```python
from build123d import *

# Parameters (mm, degrees)
F0_W     = 22
F0_H     = 35
F0_R     = 8
F1_DEPTH = 7.5
F3_DEPTH = 2
F6_DEPTH = 5
F7_R     = 2
F8_DEPTH = 35.001
F9_R     = 2.99999


# Not quite as in the source:
# - a fillet or chamfer is up to 0.001 mm smaller than in the source, because OpenCascade refuses the exact size


with BuildPart() as f1:
    # F0 (on Front) → F1 (new body, symmetric)
    with BuildSketch(Plane.XZ):
        with Locations((0, -2.5)):
            Rectangle(F0_W, F0_H)
        Circle(F0_R, mode=Mode.SUBTRACT)
    extrude(amount=F1_DEPTH, both=True)

    # F2 (on face) → F3 (cut)
    with BuildSketch(Plane(origin=(0, 0, -20), x_dir=(1, 0, 0), z_dir=(0, 0, -1))):
        with BuildLine():
            Line((2.5, 7.5), (-2.5, 7.5))
            Line((-2.5, 7.5), (-2.5, 2.5583377574))
            ThreePointArc((-2.5, 2.5583377574), (0, -3.5770227957), (2.5, 2.5583377574))
            Line((2.5, 2.5583377574), (2.5, 7.5))
        make_face()
    extrude(amount=-F3_DEPTH, mode=Mode.SUBTRACT)

    # F5 (on offset) → F6 (cut)
    with BuildSketch(Plane(origin=(0, 0, -18), x_dir=(1, 0, 0), z_dir=(0, 0, -1))):
        with BuildLine():
            Line((5, 7.5), (-5, 7.5))
            Line((-5, 7.5), (-5, 2.5583377574))
            ThreePointArc((-5, 2.5583377574), (0, -5.6165017654), (5, 2.5583377574))
            Line((5, 2.5583377574), (5, 7.5))
        make_face()
    extrude(amount=-F6_DEPTH, mode=Mode.SUBTRACT)

    # F7 (on face) → F8 (cut, through all)
    with BuildSketch(Plane.XY.offset(15)):
        Circle(F7_R)
    extrude(amount=-F8_DEPTH, mode=Mode.SUBTRACT)

    # F9 (radius 3 in the source; OpenCascade refuses exactly that, so slightly less here)
    f9_edges = [f1.edges().sort_by_distance(p)[0] for p in [
        (-11, 0, 15),
        (11, 0, 15),
        (0, -7.5, 15),
        (0, 7.5, 15),
        (11, -7.5, -2.5),
        (-11, -7.5, -2.5),
        (-11, 7.5, -2.5),
        (11, 7.5, -2.5),
        (0, 7.5, -20),
        (-6.75, -7.5, -20),
        (6.75, -7.5, -20),
        (-11, 0, -20),
        (11, 0, -20),
    ]]
    fillet(f9_edges, radius=F9_R)


solid = f1.part
```
Input: part model. Units: mm. Frame: model coordinates. A direction names the side the tool comes from. Give positions to 0.01 mm unless a question says otherwise; leave off trailing zeros. Order: outer loops, then holes, each group sorted by start corner. A loop starts at its lowest first (then second) coordinate and runs counter-clockwise, first axis right, second up. Notation, with made-up numbers: M 81,-34 L 93,-34 A20 ccw 93,-3 Z; hole C -3.75,1 d4. An arc over 180 degrees is marked long. One line per question, with ' | ' between items. Start each with the question number.
1. First-contact query: pin 1 Ø2 at (y, z) = (-4, -19.5) entering from +X; pin 2 Ø2.5 at (x, y) = (0, 0) entering from -Z; pin 3 Ø1 at (y, z) = (-4, -18.5) entering from -X; pin 4 Ø4.5 at (x, y) = (0, 0) entering from -Z. Flat tips, straight axial feed; report the tip coordinate or a pass-through.
2. Section query B-B (x = 0). Return the cut outline in (y, z).
3. Access query for faces 1 (the face through (5.29, -6.6, -19.14)), 2 (the face through (-0.161, 5.614, -15.535)), 3 (the face through (-2.5, -4, -19)), 4 (the face through (-0.119, 3.575, -19.014)). Directions: +Z, -Z, +X, -X, +Y, -Y. A direction counts if a zero-diameter tool reaches every point of the face in a straight line with its end or side. Return the directions, or none.
4. Pull-direction query (Z, two-part tool) for faces 5 (the face through (0, 7.5, -9)), 6 (the face through (-10.14, -0.06, -19.1)), 7 (the face through (-0.1, -2.5, -13)); classes: released by +Z, released by -Z, zero draft, split by the parting line, or undercut.
5. Section query C-C (y = 0). Return the cut outline in (x, z), and give its area (3 significant figures).
6. Material intervals for probe 1 along Y at (x, z) = (0, 10.5); probe 2 along Z at (x, y) = (3.5, 2.25); probe 3 along Z at (x, y) = (0, -3.5), sorted ascending. Write a range as [from, to].
7. Section query D-D (z = -12). Return the cut outline in (x, y), and give its area (3 significant figures).
Here are the results:
1) pin 1: x = 10.6 | pin 2: through | pin 3: x = -10.83 | pin 4: z = -13
2) outline: M -7.5,-13 L -2,-13 L -2,-8 L -7.5,-8 Z; M -7.5,8 L -2,8 L -2,15 L -4.5,15 A3 ccw -7.5,12 Z; M 2,-13 L 5.62,-13 L 5.62,-18 L 3.58,-18 L 3.58,-20 L 4.5,-20 A3 ccw 7.5,-17 L 7.5,-8 L 2,-8 Z; M 2,8 L 7.5,8 L 7.5,12 A3 ccw 4.5,15 L 2,15 Z
3) face 1: -Z, +X, -X, -Y | face 2: none | face 3: -Z, -Y | face 4: -Z
4) face 5: zero draft | face 6: released by -Z | face 7: undercut
5) outline: M -11,-17 A3 ccw -8,-20 L -3.58,-20 L -3.58,-18 L -5.62,-18 L -5.62,-13 L -2,-13 L -2,-7.75 A8 cw -2,7.75 L -2,15 L -8,15 A3 ccw -11,12 Z; M 2,-13 L 5.62,-13 L 5.62,-18 L 3.58,-18 L 3.58,-20 L 8,-20 A3 ccw 11,-17 L 11,12 A3 ccw 8,15 L 2,15 L 2,7.75 A8 cw 2,-7.75 Z | area: 442 mm²
6) probe 1: [-7.5, -2], [2, 7.5] | probe 2: [-20, -18], [-13, -7.19], [7.19, 15] | probe 3: [-13, -8], [8, 15]
7) outline: M -11,-4.5 A3 ccw -8,-7.5 L 8,-7.5 A3 ccw 11,-4.5 L 11,4.5 A3 ccw 8,7.5 L -8,7.5 A3 ccw -11,4.5 Z; hole C 0,0 d4 | area: 310 mm²
